```python
from build123d import *

# Parameters (mm, degrees)
F0_R     = 21.9075
F1_DEPTH = 22.225
F0_R_2   = 26.9875
F2_DEPTH = 6.35
F3_SIZE  = 3.175
F4_SIZE  = 0.8128
F6_D     = 9.525
F6_DEPTH = 19.05
F6_TIP   = 2.8615986981


with BuildPart() as f1:
    # F0 (on Top) → F1 (new body)
    with BuildSketch(Plane.XY):
        Circle(F0_R)
    extrude(amount=-F1_DEPTH)

    # F0 (on Top) → F2 (join)
    with BuildSketch(Plane.XY):
        Circle(F0_R_2)
        Circle(F0_R, mode=Mode.SUBTRACT)
        Circle(F0_R)
    extrude(amount=F2_DEPTH)

    # F3
    f3_edges = [f1.edges().sort_by_distance(p)[0] for p in [
        (-21.9075, 0, -22.225),
    ]]
    chamfer(f3_edges, length=F3_SIZE)

    # F4
    f4_edges = [f1.edges().sort_by_distance(p)[0] for p in [
        (-26.9875, 0, 0),
        (-26.9875, 0, 6.35),
    ]]
    chamfer(f4_edges, length=F4_SIZE)

    # F6
    with Locations(Plane.XY.offset(6.35)):
        with Locations((0, 0)):
            Hole(F6_D / 2, depth=F6_DEPTH)
            with Locations((0, 0, -(F6_DEPTH + F6_TIP / 2))):  # 118° drill point
                Cone(0, F6_D / 2, F6_TIP, mode=Mode.SUBTRACT)


solid = f1.part
```
Design review of the part built by this model. Coordinates are the model's own, in mm. A direction names the side the tool comes from. Coordinates: 2 decimals unless noted, no trailing zeros. Order: outer loops, then holes, each group sorted by start corner. A loop starts at its lowest first (then second) coordinate and runs counter-clockwise, first axis right, second up.
1) Take a section at B-B, the plane z = -14.5. Give the boundary of the cut face in (x, y) (1 decimal).
2) For faces 5 (the cylindrical face through (-19.89, 18.24, 3.14)), 6 (the cylindrical face through (-4.749, -21.387, -9.392)), list the 3-axis set-ups (+Z, -Z, +X, -X, +Y, -Y) from which the entire face can be reached by the end or side of a thin tool; tool diameter is ignored.
3) Take a section at A-A, the plane z = -10.5. Give the boundary of the cut face in (x, y) (1 decimal).
4) Clearance check with flat-ended pins moving along their axes: pin 1 (12 mm diameter, centred on y = -21.5, z = -4, fed in from -X); pin 2 (1.5 mm diameter, centred on y = -13, z = -14, fed in from +X); pin 3 (8 mm diameter, centred on y = 9.5, z = -13.5, fed in from -X). State where each tip first meets the part, or that it passes through.
5) Mouldability with a two-part tool opening along X and no side actions: class faces 1 (the conical face through (-0.179, -0.807, -15.065)), 2 (the conical face through (8.715, -16.756, -22.071)), 3 (the cylindrical face through (3.78, -2.9, -3.31)), 4 (the flat face through (-13.7, -17.3, 0)) as +X half, -X half, draft (parallel to the pull), parting line (faces both ways), or undercut.
6) Wall thickness on line 1 along Y through (x, z) = (0, 1); line 2 along Y through (x, z) = (0, -7.75); line 3 along Z through (x, y) = (-6, -24): over which ranges is each line inside the solid? List them lowest first.
Returned:
1. outline: circle Ø43.8 at (0, 0); hole circle Ø3.5 at (0, 0)
2. face 5: +Z, -Z
2. face 6: -Z
3. outline: circle Ø43.8 at (0, 0); hole circle Ø9.5 at (0, 0)
4. pin 1: stops at x = -20.18
4. pin 2: stops at x = 18.16
4. pin 3: stops at x = -21.21
5. face 1: undercut
5. face 2: parting line
5. face 3: undercut
5. face 4: draft
6. line 1: y = -26.99 to -4.76, 4.76 to 26.99
6. line 2: y = -21.91 to -4.76, 4.76 to 21.91
6. line 3: z = 0 to 6.35
